Verification items for this drawing (mm, ordinates from the low corner). A direction names the side the tool comes from. Coordinates: 2 decimals unless noted, no trailing zeros. Order: outer loops, then holes, each group sorted by start corner. A loop starts at its lowest first (then second) coordinate and runs counter-clockwise, first axis right, second up. Notation, with made-up numbers: M 23,-28.75 L 36,-28.75 A23 cw 36,-12.75 Z; hole C 57,38.25 d3. An arc over 180 degrees is marked long. Return JSON: item names as keys, results as strings. Group by question number.
1. Set-up check for the marked faces 1 and 2: record each of +Z, -Z, +X, -X, +Y, -Y from which the full face is reachable in a straight line by a thin tool's end or side.
2. Section check C-C, the plane z = 6. Record the cut outline in (x, y), plus the area to 3 significant figures.
3. Section check A-A, the plane y = 16.5. Record the cut outline in (x, z).
4. Section check D-D, the plane y = 28. Record the cut outline in (x, z), plus the area to 3 significant figures.
5. Gauge pin test, flat ends, axial feed: pin 1 (3 mm diameter, centred on y = 47.5, z = 43, fed in from -X); pin 2 (1.2 mm diameter, centred on x = 28.5, z = 2, fed in from -Y); pin 3 (4 mm diameter, centred on y = 16.5, z = 1.5, fed in from -X); pin 4 (9.5 mm diameter, centred on x = 23, z = 20, fed in from +Y). Record the tip position at first contact, or that the pin passes through.
6. Section check B-B, the plane x = 24. Record the cut outline in (y, z).
7. Material ranges on line 1 along X through (y, z) = (43.5, 39.5); line 2 along Y through (x, z) = (38, 30); line 3 along X through (y, z) = (3, 21.5), recorded low to high.
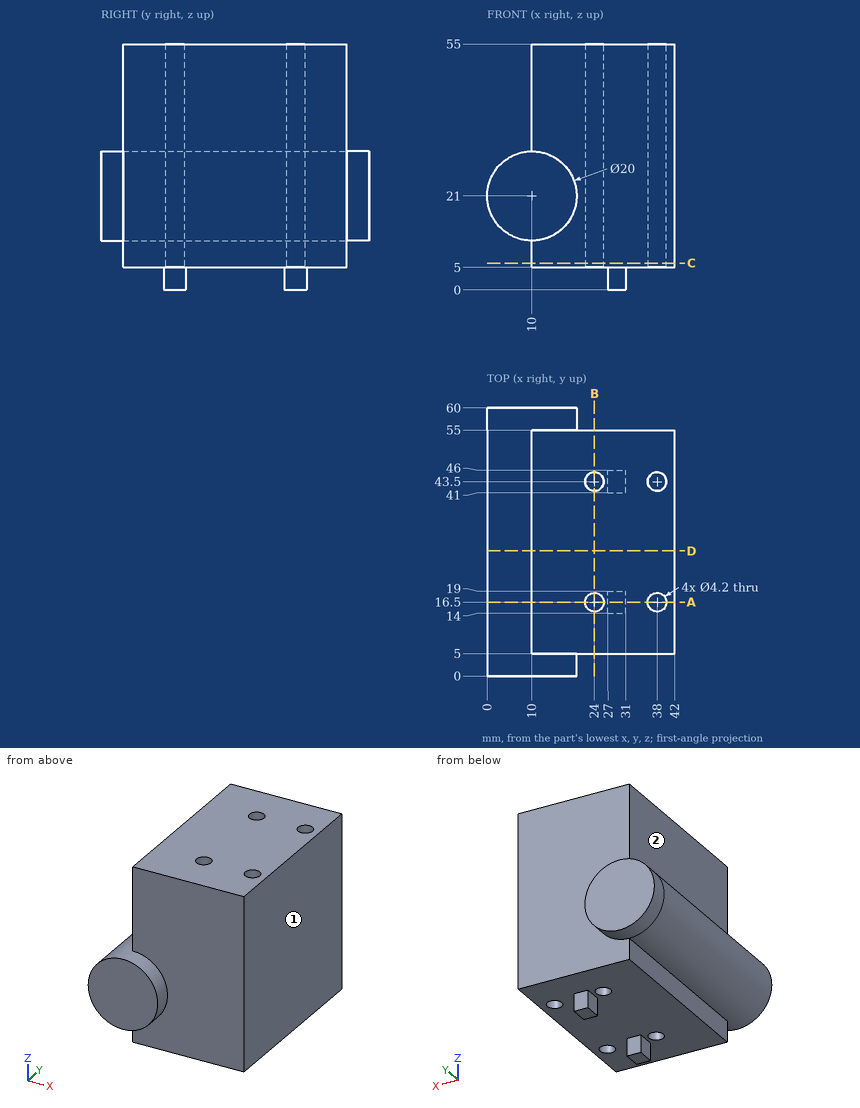
Answers follow:
{
 "1": {"face 1": "+Z, -Z, +X, +Y, -Y", "face 2": "+Z, -X, +Y, -Y"},
 "2": {"outline": "M 10,5 L 42,5 L 42,55 L 10,55 Z; hole C 24,16.5 d4.2; hole C 24,43.5 d4.2; hole C 38,16.5 d4.2; hole C 38,43.5 d4.2", "area": "1,540 mm^2"},
 "3": {"outline": "M 10,5 L 21.9,5 L 21.9,55 L 10,55 L 10,31 A10 ccw 10,11 Z; M 26.1,5 L 27,5 L 27,0 L 31,0 L 31,5 L 35.9,5 L 35.9,55 L 26.1,55 Z; M 40.1,5 L 42,5 L 42,55 L 40.1,55 Z"},
 "4": {"outline": "M 10,5 L 42,5 L 42,55 L 10,55 L 10,31 A10 ccw 10,11 Z", "area": "1,760 mm^2"},
 "5": {"pin 1": "x = 10", "pin 2": "y = 14", "pin 3": "x = 27", "pin 4": "y = 60"},
 "6": {"outline": "M 5,5 L 14.4,5 L 14.4,55 L 5,55 Z; M 18.6,5 L 41.4,5 L 41.4,55 L 18.6,55 Z; M 45.6,5 L 55,5 L 55,55 L 45.6,55 Z"},
 "7": {"line 1": "10 to 21.9, 26.1 to 35.9, 40.1 to 42", "line 2": "5 to 14.4, 18.6 to 41.4, 45.6 to 55", "line 3": "0.01 to 19.99"}
}
